from build123d import *

# Parameters (mm, degrees)
PAD029_DEPTH    = 10
PAD030_DEPTH    = 15
PAD031_DEPTH    = 15
PAD032_DEPTH    = 15
PAD033_DEPTH    = 15
SKETCH072_R     = 5
POCKET034_DEPTH = 10.001
SKETCH079_W     = 47
SKETCH079_H     = 47
PAD038_DEPTH    = 45
POCKET037_DEPTH = 35.25
SKETCH081_R     = 2.5
POCKET038_DEPTH = 10.001
SKETCH082_W     = 25
SKETCH082_H     = 9
PAD039_DEPTH    = 9.75


with BuildPart() as part:
    # Sketch067 → Pad029 (new body)
    with BuildSketch(Plane.XY):
        Polygon((-145, 28.5), (-28.5, 28.5), (-28.5, 145), (28.5, 145), (28.5, 28.5), (145, 28.5), (145, -28.5), (28.5, -28.5), (28.5, -145), (-28.5, -145), (-28.5, -28.5), (-145, -28.5), align=None)
    extrude(amount=-PAD029_DEPTH)

    # Sketch068 (on Face13 of Pad029) → Pad030 (join)
    with BuildSketch(Plane.XY):
        Polygon((-82.6, 28.5), (-82.6, -28.5), (-102.6, -28.5), (-102.6, -23.5), (-87.6, -23.5), (-87.6, 23.5), (-102.6, 23.5), (-102.6, 28.5), align=None)
    extrude(amount=PAD030_DEPTH)

    # Sketch069 (on Face7 of Pad030) → Pad031 (join)
    with BuildSketch(Plane.XY):
        Polygon((-28.5, 82.6), (28.5, 82.6), (28.5, 102.6), (23.5, 102.6), (23.5, 87.6), (-23.5, 87.6), (-23.5, 102.6), (-28.5, 102.6), align=None)
    extrude(amount=PAD031_DEPTH)

    # Sketch070 (on Face7 of Pad031) → Pad032 (join)
    with BuildSketch(Plane.XY):
        Polygon((82.6, 28.5), (102.6, 28.5), (102.6, 23.5), (87.6, 23.5), (87.6, -23.5), (102.6, -23.5), (102.6, -28.5), (82.6, -28.5), align=None)
    extrude(amount=PAD032_DEPTH)

    # Sketch071 (on Face7 of Pad032) → Pad033 (join)
    with BuildSketch(Plane.XY):
        Polygon((-28.5, -82.6), (28.5, -82.6), (28.5, -102.6), (23.5, -102.6), (23.5, -87.6), (-23.5, -87.6), (-23.5, -102.6), (-28.5, -102.6), align=None)
    extrude(amount=PAD033_DEPTH)

    # Sketch072 (on Face7 of Pad033) → Pocket034 (cut, through all)
    with BuildSketch(Plane.XY):
        with Locations((-120, 0)):
            Circle(SKETCH072_R)
        with Locations((0, 120)):
            Circle(SKETCH072_R)
        with Locations((120, 0)):
            Circle(SKETCH072_R)
        with Locations((0, -120)):
            Circle(SKETCH072_R)
    extrude(amount=-POCKET034_DEPTH, mode=Mode.SUBTRACT)

    # Sketch079 (on Face7 of Pocket034) → Pad038 (join)
    with BuildSketch(Plane.XY):
        Rectangle(SKETCH079_W, SKETCH079_H)
    extrude(amount=PAD038_DEPTH)

    # Sketch080 (on Face53 of Pad038) → Pocket037 (cut)
    with BuildSketch(Plane.XY.offset(45)):
        Polygon((-21.25, 21.25), (-12.5, 21.25), (-12.5, 23.5), (12.5, 23.5), (12.5, 21.25), (21.25, 21.25), (21.25, -21.25), (-21.25, -21.25), align=None)
    extrude(amount=-POCKET037_DEPTH, mode=Mode.SUBTRACT)

    # Sketch081 (on Face7 of Pocket037) → Pocket038 (cut, through all)
    with BuildSketch(Plane.XY):
        with Locations((0, 35.5)):
            Circle(SKETCH081_R)
    extrude(amount=-POCKET038_DEPTH, mode=Mode.SUBTRACT)

    # Sketch082 (on Face7 of Pocket038) → Pad039 (join)
    with BuildSketch(Plane.XY):
        with Locations((0, 28)):
            Rectangle(SKETCH082_W, SKETCH082_H)
    extrude(amount=PAD039_DEPTH)


solid = part.part
Model file for the job. Use its own axes, mm. A direction names the side the tool comes from. Round coordinates to 2 decimals unless told otherwise and drop trailing zeros. Loops run counter-clockwise (first coordinate to the right, second up) from the corner with the lowest first, then second, coordinate; pieces in that order, holes last.
1. Tool access for faces 4 (the flat face through (0, -86, 15)), 5 (the flat face through (23.5, -95, 7)), 6 (the flat face through (21.25, 0, 28)): list every direction of +Z, -Z, +X, -X, +Y, -Y with a clear straight run to the whole face (end or side of a thin tool).
Check values:
face 4: +Z, +X, -X, -Y
face 5: +Z, -Y
face 6: +Z
2. Mould opens along X. For faces 1 (the flat face through (-28.5, 86, -3)), 2 (the flat face through (-95, -23.5, 7)), 3 (the flat face through (-23.5, -95, 7)) say: +X half, -X half, draft (parallel to the pull), parting line (faces both ways), or undercut.
Check values:
face 1: -X half
face 2: draft
face 3: undercut
3. Band-saw the part on C-C, the plane y = 0. List the corners of the cut face in (x, z).
Check values:
outline: (-145, -10) - (-125, -10) - (-125, 0) - (-145, 0) - close; (-115, -10) - (115, -10) - (115, 0) - (87.6, 0) - (87.6, 15) - (82.6, 15) - (82.6, 0) - (23.5, 0) - (23.5, 45) - (21.25, 45) - (21.25, 9.75) - (-21.25, 9.75) - (-21.25, 45) - (-23.5, 45) - (-23.5, 0) - (-82.6, 0) - (-82.6, 15) - (-87.6, 15) - (-87.6, 0) - (-115, 0) - close; (125, -10) - (145, -10) - (145, 0) - (125, 0) - close
4. Drop flat-ended pins along their axis: P1, Ø20, axis at x = 111.5, z = 5.5, coming from the -Y side; P2, Ø1.5, axis at y = -35.5, z = -4.5, coming from the +X side; P3, Ø2, axis at y = -16.5, z = 39.5, coming from the -X side. Give the stop position or say it passes through.
Check values:
P1: stops at y = -28.5
P2: stops at x = 28.5
P3: stops at x = -23.5
5. Band-saw the part on D-D, the plane z = -4. List the corners of the cut face in (x, y), and give its area (3 significant figures).
Check values:
outline: (-145, -28.5) - (-28.5, -28.5) - (-28.5, -145) - (28.5, -145) - (28.5, -28.5) - (145, -28.5) - (145, 28.5) - (28.5, 28.5) - (28.5, 145) - (-28.5, 145) - (-28.5, 28.5) - (-145, 28.5) - close; hole circle Ø10 at (-120, 0); hole circle Ø10 at (0, -120); hole circle Ø10 at (0, 120); hole circle Ø5 at (0, 35.5); hole circle Ø10 at (120, 0)
area: 29,500 mm2
6. Wall check: probe 1 along Y at (x, z) = (0, -7); probe 2 along Y at (x, z) = (120, -2); probe 3 along Z at (x, y) = (-3.5, -92). Give the ranges that are in metal, low to high.
Check values:
probe 1: y = -145 to -125, -115 to 33, 38 to 115, 125 to 145
probe 2: y = -28.5 to -5, 5 to 28.5
probe 3: z = -10 to 0
7. Band-saw the part on A-A, the plane y = 120. List the corners of the cut face in (x, z), and give its area (3 significant figures).
Check values:
outline: (-28.5, -10) - (-5, -10) - (-5, 0) - (-28.5, 0) - close; (5, -10) - (28.5, -10) - (28.5, 0) - (5, 0) - close
area: 470 mm2
